Source: CAD feature listing. Evaluate the final solid. Frame: model axes, mm. A direction names the side the tool comes from. Round coordinates to 2 decimals unless told otherwise and drop trailing zeros. Loops run counter-clockwise (first coordinate to the right, second up) from the corner with the lowest first, then second, coordinate; pieces in that order, holes last.
Item 1: Ray query, L1, parallel to Y at x = -0.5, z = -1.5; L2, parallel to Z at x = 1, y = 17.5; L3, parallel to Y at x = -5.5, z = -25. Return the intervals inside material, ascending.
Item 2: Section query D-D on y = 20. Return loops of the section in (x, z), then the cut area to 3 significant figures.
Item 3: First-contact query: P1, Ø10, axis at x = 3.5, z = -9.5, coming from the +Y side; P2, Ø2, axis at x = -1, z = -17.5, coming from the +Y side; P3, Ø4, axis at x = 5.5, z = -9, coming from the -Y side; P4, Ø1.5, axis at x = -8, y = 17.5, coming from the -Z side. Flat tips, straight axial feed; report the tip coordinate or a pass-through.
Item 4: Section query B-B on z = -6.5. Return loops of the section in (x, y).
Item 5: Section query C-C on z = 6. Return loops of the section in (x, y), then the cut area to 3 significant figures.
Item 6: Pull-direction query (Y, two-part tool) for faces 3 (the flat face through (-0.14, 9.093, -4.563)), 4 (the flat face through (-0.14, 23.93, -12.03)), 5 (the flat face through (0.056, 2.25, -8.836)), 6 (the flat face through (-4, 0, -1)); classes: released by +Y, released by -Y, zero draft, split by the parting line, or undercut.
Item 7: Access query for faces 1 (the flat face through (0, 1, 0)), 2 (the flat face through (-10, 19, -18)). Directions: +Z, -Z, +X, -X, +Y, -Y. A direction counts if a zero-diameter tool reaches every point of the face in a straight line with its end or side. Return the directions, or none.
Item 8: Section query A-A on x = -1.25. Return loops of the section in (y, z), then the cut area to 3 significant figures.
```python
from build123d import *

# Parameters (mm, degrees)
EXTRUDE_2_DEPTH     = 4
SKETCH_5_W          = 20
SKETCH_5_H          = 32
EXTRUDE_5_DEPTH     = 20
CUT_EXTRUDE_3_DEPTH = 20


with BuildPart() as part:
    # 草图1 → 凸台-拉伸2 (new body, symmetric)
    with BuildSketch(Plane(origin=(0, 0, 0), x_dir=(0, 0, -1), z_dir=(1, 0, 0))):
        with BuildLine():
            Line((-8, 1), (7.585786438, 1))
            Line((7.585786438, 1), (27.091883092, 20.506096654))
            ThreePointArc((27.091883092, 20.506096654), (28.506096654, 20.506096654), (28.506096654, 19.091883092))
            Line((28.506096654, 19.091883092), (8.707106781, -0.707106781))
            ThreePointArc((8.707106781, -0.707106781), (8.382683432, -0.923879533), (8, -1))
            Line((8, -1), (-8, -1))
            ThreePointArc((-8, -1), (-9, 0), (-8, 1))
        make_face()
    extrude(amount=EXTRUDE_2_DEPTH, both=True)

    # 草图5 → 凸台-拉伸5 (add)
    with BuildSketch(Plane(origin=(0, -4.707106781, -4.707106781), x_dir=(1, 0, 0), z_dir=(0, -0.707106781, -0.707106781))):
        with Locations((0, -25.656854249)):
            Rectangle(SKETCH_5_W, SKETCH_5_H)
    extrude(amount=-EXTRUDE_5_DEPTH)

    # 草图6 → 切除-拉伸3 (cut)
    with BuildSketch(Plane.ZY.offset(10)):
        Polygon((2.606601718, 16.263455967), (-27.091883092, 31.819805153), (-20.02081528, 38.890872965), align=None)
    extrude(amount=-CUT_EXTRUDE_3_DEPTH, mode=Mode.SUBTRACT)


solid = part.part
```
Data:
1. L1: y = -1 to 1, 12.16 to 18.41
1. L2: z = -26.91 to 0.25
1. L3: y = 15.59 to 30.72
2. outline: (-10, -29.41) - (10, -29.41) - (10, -4.53) - (-10, -4.53) - close
2. area: 498 mm2
3. P1: stops at y = 25.22
3. P2: stops at y = 27.32
3. P3: stops at y = -1
3. P4: stops at z = -27.66
4. outline: (-10, 7.16) - (10, 7.16) - (10, 21.03) - (-10, 21.03) - close; (-4, -1) - (4, -1) - (4, 1) - (-4, 1) - close
5. outline: (-4, -1) - (4, -1) - (4, 1) - (-4, 1) - close
5. area: 16.0 mm2
6. face 3: undercut
6. face 4: released by +Y
6. face 5: undercut
6. face 6: zero draft
7. face 1: +Z, +X, -X
7. face 2: +Z, -Z, -X, +Y, -Y
8. outline: (-1, -8) arc R1 ccw to (-0.71, -8.71) - (24.75, -34.16) - (31.82, -27.09) - (16.26, 2.61) - (3.54, -10.12) - (1, -7.59) - (1, 8) arc R1 ccw to (-1, 8) - close
8. area: 522 mm2
